Geometry: final body of the model. Coordinates: model frame, mm. Face numbers are marked on the shaded views. A direction names the side the tool comes from. Coordinates: 2 decimals unless noted, no trailing zeros. Write each loop counter-clockwise with the first axis right and the second up, starting at its lowest first coordinate (ties: lowest second). Pieces come first, ordered by that corner, then holes.
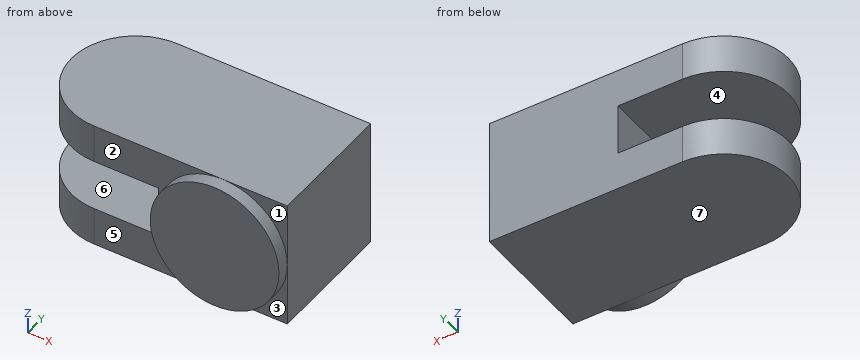
from build123d import *

# Parameters (mm, degrees)
SKETCH_1_W          = 10
SKETCH_1_H          = 10
EXTRUDE_1_DEPTH     = 10
SKETCH_2_W          = 3
SKETCH_2_H          = 10
EXTRUDE_2_DEPTH     = 10
CUT_EXTRUDE_1_DEPTH = 10
SKETCH_4_R          = 5
EXTRUDE_3_DEPTH     = 1


with BuildPart() as part:
    # 草图1 → 凸台-拉伸1 (new body)
    with BuildSketch(Plane(origin=(0, 0, 0), x_dir=(1, 0, 0), z_dir=(0, 1, 0))):
        Rectangle(SKETCH_1_W, SKETCH_1_H)
    extrude(amount=EXTRUDE_1_DEPTH)

    # 草图2 → 凸台-拉伸2 (add)
    with BuildSketch(Plane.ZY.offset(5)):
        with Locations((-3.5, 5)):
            Rectangle(SKETCH_2_W, SKETCH_2_H)
        with Locations((3.5, 5)):
            Rectangle(SKETCH_2_W, SKETCH_2_H)
    extrude(amount=EXTRUDE_2_DEPTH)

    # 草图3 → 切除-拉伸1 (cut)
    with BuildSketch(Plane.XY.offset(5)):
        with BuildLine():
            Line((-10, 10), (-17.018915749, 10))
            Line((-17.018915749, 10), (-17.018915749, 0))
            Line((-17.018915749, 0), (-10, 0))
            ThreePointArc((-10, 0), (-15, 5), (-10, 10))
        make_face()
    extrude(amount=-CUT_EXTRUDE_1_DEPTH, mode=Mode.SUBTRACT)

    # 草图4 → 凸台-拉伸3 (add)
    with BuildSketch(Plane.XZ):
        Circle(SKETCH_4_R)
    extrude(amount=EXTRUDE_3_DEPTH)


solid = part.part
Item 1: Section C-C, the plane z = 4.75. Output: boundary loops of the cut face in (x, y), plus the area to 3 significant figures.
Derived:
outline: (-10, 0) - (-1.56, 0) - (-1.56, -1) - (1.56, -1) - (1.56, 0) - (5, 0) - (5, 10) - (-10, 10) arc R5 ccw to start
area: 192 mm2
Item 2: Section B-B, the plane y = 5. Output: boundary loops of the cut face in (x, z), plus the area to 3 significant figures.
Derived:
outline: (-15, -5) - (5, -5) - (5, 5) - (-15, 5) - (-15, 2) - (-5, 2) - (-5, -2) - (-15, -2) - close
area: 160 mm2
Item 3: Section D-D, the plane x = -11.5. Output: boundary loops of the cut face in (y, z).
Derived:
outline: (0.23, -5) - (9.77, -5) - (9.77, -2) - (0.23, -2) - close; (0.23, 2) - (9.77, 2) - (9.77, 5) - (0.23, 5) - close
Item 4: Set-up query: the marked faces 1, 2, 3 and 4. Return all of +Z, -Z, +X, -X, +Y, -Y with unobstructed straight access to the full face (end or side cutting, diameter ignored); none if empty.
Derived:
face 1: +Z, +X, -Y
face 2: +Z, -X, -Y
face 3: -Z, +X, -Y
face 4: -X, +Y, -Y
Item 5: Material intervals for probe 1 along Z at (x, y) = (-11, 5); probe 2 along X at (y, z) = (1.75, 0.5); probe 3 along Y at (x, z) = (-8.25, 4.5), sorted ascending.
Derived:
probe 1: z = -5 to -2, 2 to 5
probe 2: x = -5 to 5
probe 3: y = 0 to 10
Item 6: Pull-direction query (Z, two-part tool) for the marked faces 5, 6 and 7; classes: released by +Z, released by -Z, zero draft, split by the parting line, or undercut.
Derived:
face 5: zero draft
face 6: undercut
face 7: released by -Z
Item 7: Section A-A, the plane x = -8.5. Output: boundary loops of the cut face in (y, z), plus the area to 3 significant figures.
Derived:
outline: (0, -5) - (10, -5) - (10, -2) - (0, -2) - close; (0, 2) - (10, 2) - (10, 5) - (0, 5) - close
area: 60.0 mm2
Item 8: Pin query (flat end, axial travel): pin 1 (2 mm diameter, centred on y = 5, z = -0.5, fed in from -X); pin 2 (1 mm diameter, centred on y = 3.5, z = -4, fed in from -X); pin 3 (1.5 mm diameter, centred on y = 2, z = -1.5, fed in from -X). Return the tip coordinate at first contact, or that it passes through.
Derived:
pin 1: stops at x = -5
pin 2: stops at x = -14.9
pin 3: stops at x = -14.36
